Part model, mm, in its own coordinate system. Face numbers are marked on the shaded views. A direction names the side the tool comes from. Give positions to 0.01 mm unless a question says otherwise; leave off trailing zeros. Loops run counter-clockwise (first coordinate to the right, second up) from the corner with the lowest first, then second, coordinate; pieces in that order, holes last. Notation, with made-up numbers: (65.5, 22.5) -> (89.5, 22.5) arc R32 cw to (89.5, 57.5) -> close; hole circle Ø1 at (47.5, 47). An arc over 180 degrees is marked (long way). Write item = value, one per line.
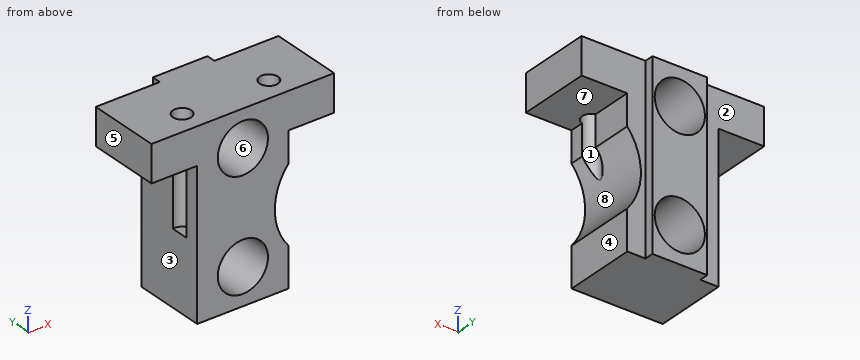
from build123d import *

# Parameters (mm, degrees)
BOSS_EXTRUDE1_DEPTH = 8
SKETCH5_W           = 6
SKETCH5_H           = 20
BOSS_EXTRUDE2_DEPTH = 1
SKETCH6_R           = 6.5
CUT_EXTRUDE3_DEPTH  = 10
SKETCH2_R           = 2.75
CUT_EXTRUDE1_DEPTH  = 10
SKETCH3_R           = 1
CUT_EXTRUDE2_DEPTH  = 12


with BuildPart() as part:
    # Sketch1 → Boss-Extrude1 (new body)
    with BuildSketch(Plane(origin=(0, 0, 0), x_dir=(1, 0, 0), z_dir=(0, 1, 0))):
        Polygon((-10, 0), (10, 0), (10, 4), (5, 4), (5, 20), (-5, 20), (-5, 4), (-10, 4), align=None)
    extrude(amount=BOSS_EXTRUDE1_DEPTH)

    # Sketch5 → Boss-Extrude2 (add)
    with BuildSketch(Plane(origin=(0, 8, 0), x_dir=(1, 0, 0), z_dir=(0, 1, 0))):
        with Locations((0, 10)):
            Rectangle(SKETCH5_W, SKETCH5_H)
    extrude(amount=BOSS_EXTRUDE2_DEPTH)

    # Sketch6 → Cut-Extrude3 (cut, through all)
    with BuildSketch(Plane.XZ):
        with Locations((10, -11.5)):
            Circle(SKETCH6_R)
    extrude(amount=-CUT_EXTRUDE3_DEPTH, mode=Mode.SUBTRACT)

    # Sketch2 → Cut-Extrude1 (cut, through all)
    with BuildSketch(Plane.XZ):
        with Locations((0, -4)):
            Circle(SKETCH2_R)
        with Locations((0, -16)):
            Circle(SKETCH2_R)
    extrude(amount=-CUT_EXTRUDE1_DEPTH, mode=Mode.SUBTRACT)

    # Sketch3 → Cut-Extrude2 (cut)
    with BuildSketch(Plane.XY):
        with Locations((-4.75, 2.5)):
            Circle(SKETCH3_R)
        with Locations((4.75, 2.5)):
            Circle(SKETCH3_R)
    extrude(amount=-CUT_EXTRUDE2_DEPTH, mode=Mode.SUBTRACT)


solid = part.part
1) Slice it at A-A, the plane y = 2.5. List the corners of the cut face in (x, z), and give its area (3 significant figures).
Resolved:
outline = (-10, -4) -> (-5.75, -4) -> (-5.75, 0) -> (-10, 0) -> close; (-5, -20) -> (5, -20) -> (5, -15.65) arc R6.5 cw to (3.75, -9.71) -> (3.75, 0) -> (-3.75, 0) -> (-3.75, -12) -> (-5, -12) -> close; (5.75, -4) -> (10, -4) -> (10, 0) -> (5.75, 0) -> close; hole circle Ø5.5 at (0, -16); hole circle Ø5.5 at (0, -4)
area = 153 mm²
2) Drill centre lines: line 1 along Z through (x, y) = (0, 6.5); line 2 along Z through (x, y) = (-2, 2.5); line 3 along Z through (x, y) = (-4.5, 1.75). Where is each one in solid material? Low to high. Write a range as [from, to].
Resolved:
line_1 = [-20, -18.75], [-13.25, -6.75], [-1.25, 0]
line_2 = [-20, -17.89], [-14.11, -5.89], [-2.11, 0]
line_3 = [-20, -12]
3) Drop flat-ended pins along their axis: P1, Ø3, axis at y = 2, z = -13, coming from the +X side; P2, Ø1, axis at y = 1.5, z = -9, coming from the -X side; P3, Ø1, axis at y = 6, z = -16, coming from the +X side. Give the stop position or say it passes through.
Resolved:
P1 = 4.23
P2 = -5
P3 = 5
4) Slice it at B-B, the plane z = -2. List the corners of the cut face in (x, y), and give its area (3 significant figures).
Resolved:
outline = (-10, 0) -> (-1.89, 0) -> (-1.89, 9) -> (-3, 9) -> (-3, 8) -> (-10, 8) -> close; (1.89, 0) -> (10, 0) -> (10, 8) -> (3, 8) -> (3, 9) -> (1.89, 9) -> close; hole circle Ø2 at (-4.75, 2.5); hole circle Ø2 at (4.75, 2.5)
area = 126 mm²
5) Which spindle directions (+Z, -Z, +X, -X, +Y, -Y) get a long thin tool onto all of the face, cutting with end or side? Do the marked faces 1, 2, 3 and 4. Say none if no direction does.
Resolved:
face_1 = +Z
face_2 = +Z, -Z, -X, +Y
face_3 = -Z, -X, +Y, -Y
face_4 = -Z, +X, +Y, -Y
6) Slice it at C-C, the plane x = 0. List the corners of the cut face in (y, z), and give its area (3 significant figures).
Resolved:
outline = (0, -20) -> (9, -20) -> (9, -18.75) -> (0, -18.75) -> close; (0, -13.25) -> (9, -13.25) -> (9, -6.75) -> (0, -6.75) -> close; (0, -1.25) -> (9, -1.25) -> (9, 0) -> (0, 0) -> close
area = 81.0 mm²
7) Slice it at D-D, the plane z = -15.25. List the corners of the cut face in (x, y), and give its area (3 significant figures).
Resolved:
outline = (-5, 0) -> (-2.65, 0) -> (-2.65, 9) -> (-3, 9) -> (-3, 8) -> (-5, 8) -> close; (2.65, 0) -> (4.69, 0) -> (4.69, 8) -> (3, 8) -> (3, 9) -> (2.65, 9) -> close
area = 35.9 mm²
8) Pull direction Z, two halves, no side cores. Call the marked faces 5, 6, 7 and 8: pulls with the +Z half, pulls with the -Z half, needs draft (parallel to the pull), parting line crosses it, or undercut.
Resolved:
face_5 = needs draft
face_6 = undercut
face_7 = pulls with the -Z half
face_8 = undercut
